```python
from build123d import *

# Parameters (mm, degrees)
SALIENTE_EXTRUIR1_DEPTH = 60
CROQUIS2_R              = 2.75
CORTAR_EXTRUIR1_DEPTH   = 91.691785736
CROQUIS4_R              = 6
CORTAR_EXTRUIR2_DEPTH   = 73
CROQUIS5_W              = 41
CROQUIS5_H              = 21
CORTAR_EXTRUIR3_DEPTH   = 100.924971854
CROQUIS6_R              = 2.3
CORTAR_EXTRUIR4_DEPTH   = 100.924971854
CROQUIS7_W              = 3
CROQUIS7_H              = 3
CORTAR_EXTRUIR5_DEPTH   = 90.269255626
REDONDEO3_R             = 1.5


with BuildPart() as part:
    # Croquis1 → Saliente-Extruir1 (new body)
    with BuildSketch(Plane.XY):
        Polygon((0, 0), (0, -7), (-1, -7), (-1, -13), (0, -13), (0, -20), (79, -20), (79, -12), (14, -12), (14, 0), align=None)
    extrude(amount=SALIENTE_EXTRUIR1_DEPTH)

    # Croquis2 → Cortar-Extruir1 (cut, through all)
    with BuildSketch(Plane(origin=(14, 0, 0), x_dir=(0, 0, -1), z_dir=(1, 0, 0))):
        with Locations((-50, -10)):
            Circle(CROQUIS2_R)
        with Locations((-10, -10)):
            Circle(CROQUIS2_R)
    extrude(amount=-CORTAR_EXTRUIR1_DEPTH, mode=Mode.SUBTRACT)

    # Croquis4 → Cortar-Extruir2 (cut)
    with BuildSketch(Plane(origin=(79, 0, 0), x_dir=(0, 0, -1), z_dir=(1, 0, 0))):
        with Locations((-50, -10)):
            Circle(CROQUIS4_R)
        with Locations((-10, -10)):
            Circle(CROQUIS4_R)
    extrude(amount=-CORTAR_EXTRUIR2_DEPTH, mode=Mode.SUBTRACT)

    # Croquis5 → Cortar-Extruir3 (cut, through all)
    with BuildSketch(Plane(origin=(0, -12, 0), x_dir=(1, 0, 0), z_dir=(0, 1, 0))):
        with Locations((46.5, -30)):
            Rectangle(CROQUIS5_W, CROQUIS5_H)
    extrude(amount=-CORTAR_EXTRUIR3_DEPTH, mode=Mode.SUBTRACT)

    # Croquis6 → Cortar-Extruir4 (cut, through all)
    with BuildSketch(Plane(origin=(0, -12, 0), x_dir=(1, 0, 0), z_dir=(0, 1, 0))):
        with Locations(Location((22.25, -25.25, 0), (0, 0, 180))):
            Circle(CROQUIS6_R)
        with Locations(Location((22.25, -34.75, 0), (0, 0, 180))):
            Circle(CROQUIS6_R)
        with Locations(Location((70.75, -25.25, 0), (0, 0, 180))):
            Circle(CROQUIS6_R)
        with Locations(Location((70.75, -34.75, 0), (0, 0, 180))):
            Circle(CROQUIS6_R)
    extrude(amount=-CORTAR_EXTRUIR4_DEPTH, mode=Mode.SUBTRACT)

    # Croquis7 → Cortar-Extruir5 (cut, through all)
    with BuildSketch(Plane(origin=(14, -12, 60), x_dir=(1, 0, 0), z_dir=(0, 1, 0))):
        with Locations((54.5, 30)):
            Rectangle(CROQUIS7_W, CROQUIS7_H)
    extrude(amount=-CORTAR_EXTRUIR5_DEPTH, mode=Mode.SUBTRACT)

    # Redondeo3
    redondeo3_edges = [part.edges().sort_by_distance(p)[0] for p in [
        (70, -16, 31.5),
        (70, -16, 28.5),
    ]]
    fillet(redondeo3_edges, radius=REDONDEO3_R - 0.0001)  # a hair under: the kernel refuses the full size
    redondeo3_2_edges = [part.edges().sort_by_distance(p)[0] for p in [
        (67, -16, 28.5),
        (67, -16, 31.5),
    ]]
    fillet(redondeo3_2_edges, radius=REDONDEO3_R)


solid = part.part
```
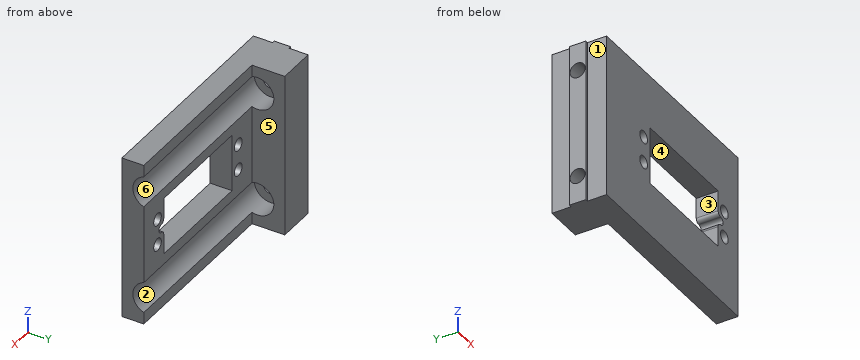
For this review, take the finished solid that the model builds, in its own axes (mm). Face numbers are marked on the shaded views. A direction names the side the tool comes from. Coordinates: 2 decimals unless noted, no trailing zeros. Loops run counter-clockwise (first coordinate to the right, second up) from the corner with the lowest first, then second, coordinate; pieces in that order, holes last. Notation, with made-up numbers: (31.5, -20.5) - (65.5, -20.5) arc R37 cw to (65.5, 18.5) - close; hole circle Ø11 at (24, -38.5). An arc over 180 degrees is marked (long way). Use one line per item in the form item = value. Start each with the question number.
1) For pin 1 (9.5 mm diameter, centred on y = -10, z = 10, fed in from +X); pin 2 (4 mm diameter, centred on y = -17.5, z = 36.5, fed in from -X); pin 3 (9.5 mm diameter, centred on y = -3, z = 32.5, fed in from +X), all flat-tipped, find the tip position at first contact; note any pin that passes through.
2) For the marked faces 4, 5 and 6, list the 3-axis set-ups (+Z, -Z, +X, -X, +Y, -Y) from which the entire face can be reached by the end or side of a thin tool; tool diameter is ignored.
3) Take a section at B-B (z = 38). State the section outline as (x, y) points.
4) Draft analysis for pull direction X (two halves, no side actions). For the marked faces 1, 2 and 3, state which applies: released by +X, released by -X, zero draft, split by the parting line, or undercut.
5) Take a section at A-A (x = 42). State the section outline as (y, z) points.
6) Take a section at D-D (x = 22.25). State the section outline as (y, z) points.
7) Take a section at C-C (y = -17.5). State how many separate pieces and enclosed holes the cut face has, plus the area to 3 significant figures.
8) To check wall thickness, follow probe 1 along Z at (x, y) = (70.75, -18); probe 2 along Z at (x, y) = (50, -18); probe 3 along Z at (x, y) = (12, -11.5). State the ranges of each line that lie inside material, in increasing order. Write a range as from..to.
From the geometry:
q1.pin_1 = 6
q1.pin_2 = 0
q1.pin_3 = 14
q2.face_4 = +Y, -Y
q2.face_5 = +Z, -Z, +X, +Y
q2.face_6 = +X
q3.outline = (-1, -13) - (0, -13) - (0, -20) - (26, -20) - (26, -12) - (14, -12) - (14, 0) - (0, 0) - (0, -7) - (-1, -7) - close; (67, -20) - (79, -20) - (79, -12) - (67, -12) - close
q4.face_1 = released by -X
q4.face_2 = zero draft
q4.face_3 = undercut
q5.outline = (-20, 0) - (-12, 0) - (-12, 4.34) arc R6 cw to (-12, 15.66) - (-12, 19.5) - (-20, 19.5) - close; (-20, 40.5) - (-12, 40.5) - (-12, 44.34) arc R6 cw to (-12, 55.66) - (-12, 60) - (-20, 60) - close
q6.outline = (-20, 0) - (-12, 0) - (-12, 4.34) arc R6 cw to (-12, 15.66) - (-12, 22.95) - (-20, 22.95) - close; (-20, 27.55) - (-12, 27.55) - (-12, 32.45) - (-20, 32.45) - close; (-20, 37.05) - (-12, 37.05) - (-12, 44.34) arc R6 cw to (-12, 55.66) - (-12, 60) - (-20, 60) - close
q7.separate_pieces = 1
q7.enclosed_holes = 5
q7.area = 3,800 mm2
q8.probe_1 = 0..22.95, 27.55..32.45, 37.05..60
q8.probe_2 = 0..19.5, 40.5..60
q8.probe_3 = 0..4.19, 15.81..44.19, 55.81..60
